Can you work these out from the model? Positions are in its coordinate system, mm. Give positions to 0.01 mm unless a question says otherwise; leave off trailing zeros. Write each loop counter-clockwise with the first axis right and the second up, starting at its lowest first coordinate (ties: lowest second). Pieces come first, ordered by that corner, then holes.
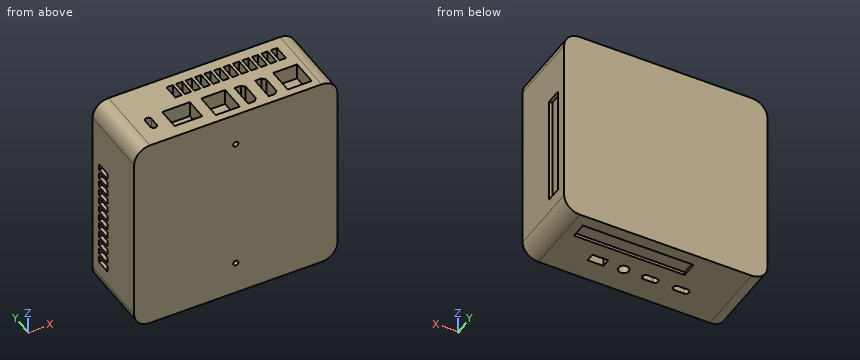
from build123d import *

# Parameters (mm, degrees)
SKETCH1_W                                     = 128.5
SKETCH1_H                                     = 127
GABARYT_DEPTH                                 = 47
SKETCH2_W                                     = 17.5
SKETCH2_H                                     = 14
SKETCH2_W_2                                   = 15.2
SKETCH2_H_2                                   = 16.5
PORTY_USBC_ETHERNET_2XUSBA_HDMI_HDMI_2X_DEPTH = 10
SKETCH3_W                                     = 4
SKETCH3_H                                     = 10
VENTS_OUTLET_1_DEPTH                          = 10
SKETCH4_W                                     = 4
SKETCH4_H                                     = 10
VENTS_OUTLET_2_DEPTH                          = 10
VENTS_START                                   = -127
SKETCH3_3_W                                   = 70
SKETCH3_3_H                                   = 10
VENTS_INLET_1_DEPTH                           = 2
VENTS_START_2                                 = -128.5
SKETCH4_3_W                                   = 70
SKETCH4_3_H                                   = 10
VENTS_INLET_2_DEPTH                           = 2
SKETCH5_R                                     = 3.25
SKETCH5_W                                     = 10
SKETCH5_H                                     = 5.5
PORTY_ON_AUDIOJACK_USBC_USBC_DEPTH            = 10
TAP_DRILL_FOR_M4_TAP1_D                       = 3.3
TAP_DRILL_FOR_M4_TAP1_DEPTH                   = 6
TAP_DRILL_FOR_M4_TAP1_TIP                     = 0.991420021
FILLET1_R                                     = 10


with BuildPart() as part:
    # Sketch1 → gabaryt (new body)
    with BuildSketch(Plane(origin=(0, 0, 0), x_dir=(1, 0, 0), z_dir=(0, 1, 0))):
        with Locations((64.25, 63.5)):
            Rectangle(SKETCH1_W, SKETCH1_H)
    extrude(amount=GABARYT_DEPTH)

    # Sketch2 → porty (usbc/ethernet/2xUSBa/hdmi/hdmi/2xUSBa) (cut)
    with BuildSketch(Plane.XY):
        with BuildLine():
            Line((22, 19.6), (22, 14))
            ThreePointArc((22, 14), (20, 12), (18, 14))
            Line((18, 14), (18, 19.6))
            ThreePointArc((18, 19.6), (20, 21.6), (22, 19.6))
        make_face()
        Polygon((75, 20.7), (75, 5.2), (79, 5.2), (81, 7.2), (81, 18.7), (79, 20.7), align=None)
        with Locations((38.75, 15)):
            Rectangle(SKETCH2_W, SKETCH2_H)
        with Locations((62.1, 13.45)):
            Rectangle(SKETCH2_W_2, SKETCH2_H_2)
        Polygon((88, 20.7), (88, 5.2), (92, 5.2), (94, 7.2), (94, 18.7), (92, 20.7), align=None)
        with Locations((107.6, 13.45)):
            Rectangle(SKETCH2_W_2, SKETCH2_H_2)
    extrude(amount=-PORTY_USBC_ETHERNET_2XUSBA_HDMI_HDMI_2X_DEPTH, mode=Mode.SUBTRACT)

    # Sketch3 → vents outlet 1 (cut)
    with BuildSketch(Plane.XY):
        with Locations((44.5, 34.5)):
            Rectangle(SKETCH3_W, SKETCH3_H)
        with Locations((50.5, 34.5)):
            Rectangle(SKETCH3_W, SKETCH3_H)
        with Locations((56.5, 34.5)):
            Rectangle(SKETCH3_W, SKETCH3_H)
        with Locations((62.5, 34.5)):
            Rectangle(SKETCH3_W, SKETCH3_H)
        with Locations((68.5, 34.5)):
            Rectangle(SKETCH3_W, SKETCH3_H)
        with Locations((74.5, 34.5)):
            Rectangle(SKETCH3_W, SKETCH3_H)
        with Locations((80.5, 34.5)):
            Rectangle(SKETCH3_W, SKETCH3_H)
        with Locations((86.5, 34.5)):
            Rectangle(SKETCH3_W, SKETCH3_H)
        with Locations((92.5, 34.5)):
            Rectangle(SKETCH3_W, SKETCH3_H)
        with Locations((98.5, 34.5)):
            Rectangle(SKETCH3_W, SKETCH3_H)
        with Locations((104.5, 34.5)):
            Rectangle(SKETCH3_W, SKETCH3_H)
        with Locations((110.5, 34.5)):
            Rectangle(SKETCH3_W, SKETCH3_H)
    extrude(amount=-VENTS_OUTLET_1_DEPTH, mode=Mode.SUBTRACT)

    # Sketch4 → vents outlet 2 (cut)
    with BuildSketch(Plane.ZY):
        with Locations((-106, 35)):
            Rectangle(SKETCH4_W, SKETCH4_H)
        with Locations((-100, 35)):
            Rectangle(SKETCH4_W, SKETCH4_H)
        with Locations((-94, 35)):
            Rectangle(SKETCH4_W, SKETCH4_H)
        with Locations((-88, 35)):
            Rectangle(SKETCH4_W, SKETCH4_H)
        with Locations((-82, 35)):
            Rectangle(SKETCH4_W, SKETCH4_H)
        with Locations((-76, 35)):
            Rectangle(SKETCH4_W, SKETCH4_H)
        with Locations((-70, 35)):
            Rectangle(SKETCH4_W, SKETCH4_H)
        with Locations((-64, 35)):
            Rectangle(SKETCH4_W, SKETCH4_H)
        with Locations((-58, 35)):
            Rectangle(SKETCH4_W, SKETCH4_H)
        with Locations((-52, 35)):
            Rectangle(SKETCH4_W, SKETCH4_H)
        with Locations((-46, 35)):
            Rectangle(SKETCH4_W, SKETCH4_H)
        with Locations((-40, 35)):
            Rectangle(SKETCH4_W, SKETCH4_H)
    extrude(amount=-VENTS_OUTLET_2_DEPTH, mode=Mode.SUBTRACT)

    # Sketch3<3> → vents inlet 1 (cut)
    with BuildSketch(Plane.XY.offset(VENTS_START)):
        with Locations((77.5, 34.5)):
            Rectangle(SKETCH3_3_W, SKETCH3_3_H)
    extrude(amount=VENTS_INLET_1_DEPTH, mode=Mode.SUBTRACT)

    # Sketch4<3> → vents inlet 2 (cut)
    with BuildSketch(Plane.ZY.offset(VENTS_START_2)):
        with Locations((-73, 35)):
            Rectangle(SKETCH4_3_W, SKETCH4_3_H)
    extrude(amount=VENTS_INLET_2_DEPTH, mode=Mode.SUBTRACT)

    # Sketch5 → porty (on/audiojack/USBc/USBc) (cut)
    with BuildSketch(Plane(origin=(0, 0, -127), x_dir=(-1, 0, 0), z_dir=(0, 0, -1))):
        with Locations((-74.25, 17.25)):
            Circle(SKETCH5_R)
        with Locations((-90.5, 17.25)):
            Rectangle(SKETCH5_W, SKETCH5_H)
        with BuildLine():
            Line((-60.5, 19.25), (-54.5, 19.25))
            ThreePointArc((-54.5, 19.25), (-52.5, 17.25), (-54.5, 15.25))
            Line((-54.5, 15.25), (-60.5, 15.25))
            ThreePointArc((-60.5, 15.25), (-62.5, 17.25), (-60.5, 19.25))
        make_face()
        with BuildLine():
            Line((-41, 19.25), (-35, 19.25))
            ThreePointArc((-35, 19.25), (-33, 17.25), (-35, 15.25))
            Line((-35, 15.25), (-41, 15.25))
            ThreePointArc((-41, 15.25), (-43, 17.25), (-41, 19.25))
        make_face()
    extrude(amount=-PORTY_ON_AUDIOJACK_USBC_USBC_DEPTH, mode=Mode.SUBTRACT)

    # Tap Drill for M4 Tap1
    with Locations(Plane(origin=(0, 0, 0), x_dir=(-1, 0, 0), z_dir=(0, -1, 0))):
        with Locations((-64.25, 106), (-64.25, 21)):
            Hole(TAP_DRILL_FOR_M4_TAP1_D / 2, depth=TAP_DRILL_FOR_M4_TAP1_DEPTH)
            with Locations((0, 0, -(TAP_DRILL_FOR_M4_TAP1_DEPTH + TAP_DRILL_FOR_M4_TAP1_TIP / 2))):  # 118° drill point
                Cone(0, TAP_DRILL_FOR_M4_TAP1_D / 2, TAP_DRILL_FOR_M4_TAP1_TIP, mode=Mode.SUBTRACT)

    # Fillet1
    fillet1_edges = [part.edges().sort_by_distance(p)[0] for p in [
        (0, 23.5, -127),
        (128.5, 23.5, -127),
        (128.5, 23.5, 0),
        (0, 23.5, 0),
    ]]
    fillet(fillet1_edges, radius=FILLET1_R)


solid = part.part
(1) Will these pins go through, and if not, where does the flat tip stop? P1, Ø8, axis at y = 34, z = -6, coming from the +X side; P2, Ø7.5, axis at x = 60, y = 14, coming from the +Z side; P3, Ø8, axis at y = 34.5, z = -78, coming from the +X side; P4, Ø8, axis at y = 13.5, z = -5.5, coming from the -X side.
Returned:
P1: stops at x = 128.5
P2: stops at z = -10
P3: stops at x = 126.5
P4: stops at x = 0.01
(2) If I drill on L1, parallel to Z at x = 64, y = 2; L2, parallel to Y at x = 74.25, z = -120.5; L3, parallel to X at y = 17, z = -118, over which ranges is the centre line in solid material (lowest first)?
Returned:
L1: z = -127 to -107.63, -104.37 to -22.63, -19.37 to 0
L2: y = 0 to 14, 20.5 to 47
L3: x = 0.05 to 33.02, 42.98 to 52.52, 62.48 to 71.01, 77.49 to 85.5, 95.5 to 128.45
(3) Imagine slicing it at A-A, the plane z = -88. Write out the boundary of the cut face in (x, y).
Returned:
outline: (0, 0) - (128.5, 0) - (128.5, 30) - (126.5, 30) - (126.5, 40) - (128.5, 40) - (128.5, 47) - (0, 47) - (0, 40) - (10, 40) - (10, 30) - (0, 30) - close
